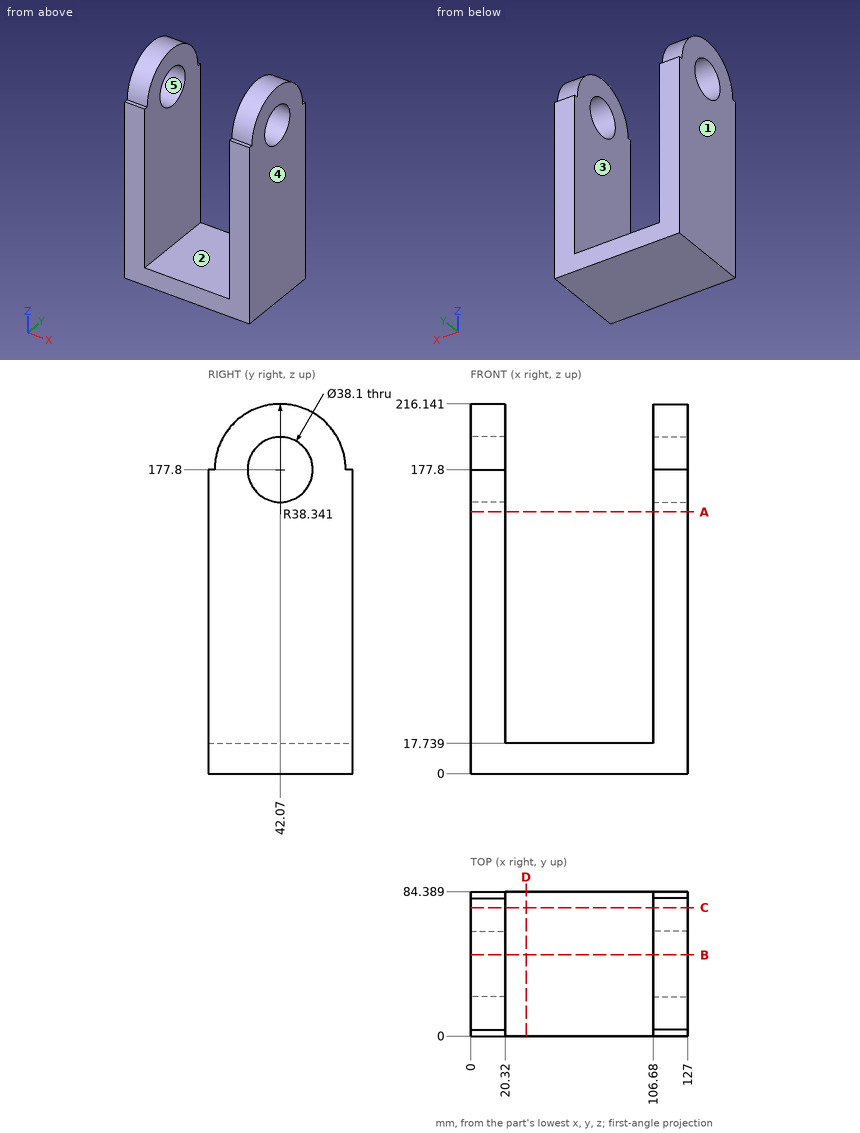
Here's the drawing with two shaded views (mm, measured from the low corner). I have some questions. A direction names the side the tool comes from. Coordinates: 2 decimals unless noted, no trailing zeros. Write each loop counter-clockwise with the first axis right and the second up, starting at its lowest first coordinate (ties: lowest second). Pieces come first, ordered by that corner, then holes. Notation, with made-up numbers: M 55.5,16.25 L 70.5,16.25 A21 ccw 70.5,48.25 Z; hole C 47.25,33 d10. An arc over 180 degrees is marked long. Answer as CSV lines item,"result". Start each with the question number.
1) For P1, Ø4, axis at x = 78, y = 70.5, coming from the +Z side; P2, Ø2, axis at x = 13, y = 82.5, coming from the +Z side; P3, Ø23, axis at y = 42.07, z = 177.8, coming from the -X side, each with a flat end and sliding along its axis, tell me the tip position at first contact or that it passes through.
2) I want a section at D-D, the plane x = 32.5. Please give me the cut outline in (y, z), and give its area (3 significant figures).
3) I want a section at B-B, the plane y = 47.5. Please give me the cut outline in (x, z) (1 decimal), and give its area (3 significant figures).
4) For the marked faces 1 and 2, which set-ups out of +Z, -Z, +X, -X, +Y, -Y let a thin tool reach every point of the face, with its end or its side?
5) We'd pull the mould along X, two halves only. Please class the marked faces 3, 4 and 5: +X half, -X half, draft (parallel to the pull), parting line (faces both ways), or undercut.
6) I want a section at C-C, the plane y = 75. Please give me the cut outline in (x, z).
7) Please list where these lines run through material, in increasing order: line 1 (X direction, y = 16, z = 21.5); line 2 (Z direction, x = 48.5, y = 23); line 3 (Z direction, x = 9, y = 35.5) (1 decimal). Write a range as from..to.
8) I want a section at A-A, the plane z = 153. Please give me the cut outline in (x, y), and give its area (3 significant figures).
Data:
1,P1,"stops at z = 17.74"
1,P2,"stops at z = 177.8"
1,P3,"passes through"
2,outline,"M 0,0 L 84.39,0 L 84.39,17.74 L 0,17.74 Z"
2,area,"1,500 mm^2"
3,outline,"M 0,0 L 127,0 L 127,159.5 L 106.7,159.5 L 106.7,17.7 L 20.3,17.7 L 20.3,159.5 L 0,159.5 Z; M 0,196.1 L 20.3,196.1 L 20.3,215.8 L 0,215.8 Z; M 106.7,196.1 L 127,196.1 L 127,215.8 L 106.7,215.8 Z"
3,area,"8,820 mm^2"
4,face 1,"+Z, -Z, -X, +Y, -Y"
4,face 2,"+Z, +Y, -Y"
5,face 3,"undercut"
5,face 4,"+X half"
5,face 5,"draft"
6,outline,"M 0,0 L 127,0 L 127,197.44 L 106.68,197.44 L 106.68,17.74 L 20.32,17.74 L 20.32,197.44 L 0,197.44 Z"
7,line 1,"x = 0..20.32, 106.68..127"
7,line 2,"z = 0..17.74"
7,line 3,"z = 0..159.9, 195.7..215.6"
8,outline,"M 0,0 L 20.32,0 L 20.32,84.39 L 0,84.39 Z; M 106.68,0 L 127,0 L 127,84.39 L 106.68,84.39 Z"
8,area,"3,430 mm^2"
